Job drawing, mm, ordinate dimensions from the low corner. One solid piece. A direction names the side the tool comes from. Round coordinates to 2 decimals unless told otherwise and drop trailing zeros. Order: outer loops, then holes, each group sorted by start corner. A loop starts at its lowest first (then second) coordinate and runs counter-clockwise, first axis right, second up. Notation, with made-up numbers: (-1, 70.5) -> (42, 70.5) arc R22 cw to (42, 104.5) -> close; hole circle Ø3 at (1.5, -36). An arc over 180 degrees is marked (long way). Use CSV: the item, a comma, the result in double quotes.
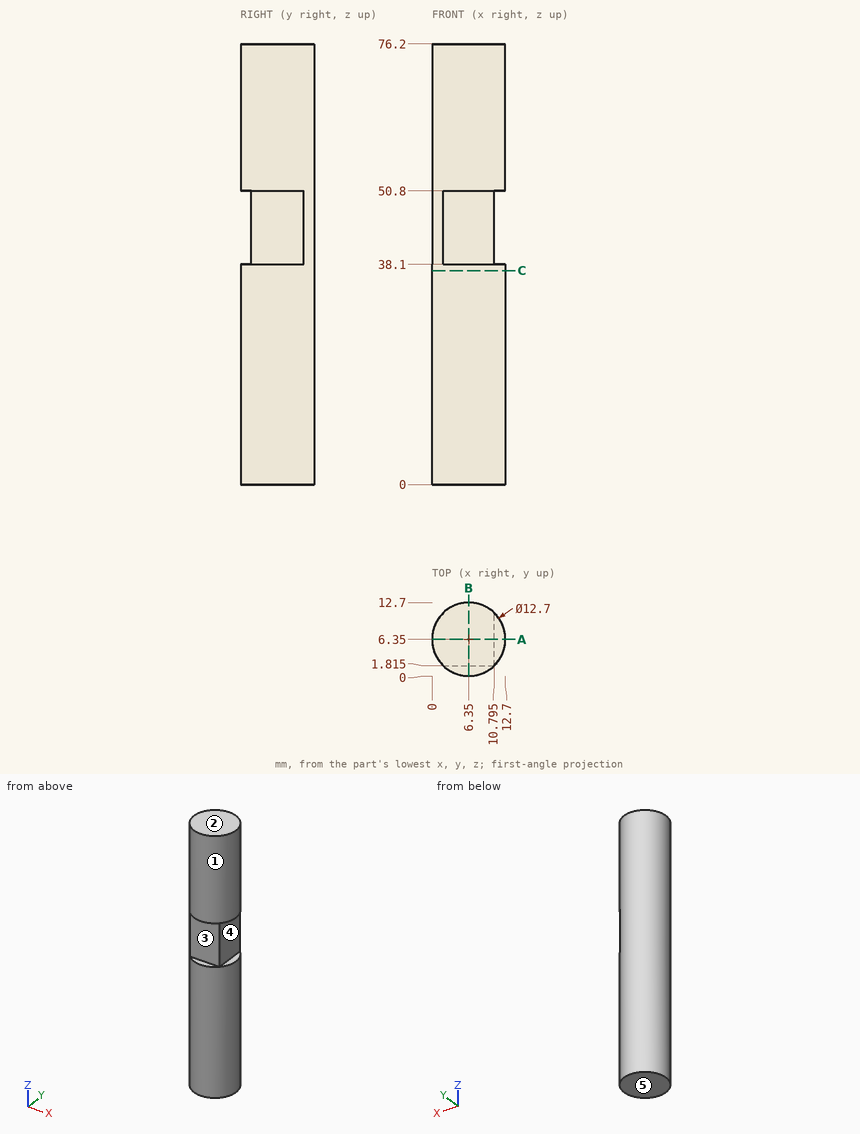
(1) Pull direction Z, two halves, no side cores. Call the marked faces 1, 2 and 3: released by +Z, released by -Z, zero draft, split by the parting line, or undercut.
Reply:
face 1,"zero draft"
face 2,"released by +Z"
face 3,"undercut"
(2) Cut at A-A, the plane y = 6.35. Give the cut face in (x, z) (3 decimals).
Reply:
outline,"(0, 0) -> (12.7, 0) -> (12.7, 38.1) -> (10.795, 38.1) -> (10.795, 50.8) -> (12.7, 50.8) -> (12.7, 76.2) -> (0, 76.2) -> close"
(3) Drop flat-ended pins along their axis: P1, Ø3, axis at y = 2.5, z = 30.5, coming from the -X side; P2, Ø4, axis at y = 3.5, z = 43.5, coming from the -X side; P3, Ø3, axis at y = 3, z = 13.5, coming from the +X side. Give the stop position or say it passes through.
Reply:
P1,"x = 0.45"
P2,"x = 0.06"
P3,"x = 12.42"
(4) Cut at C-C, the plane z = 37. Give the cut face in (x, y).
Reply:
outline,"circle Ø12.7 at (6.35, 6.35)"
(5) Cut at B-B, the plane x = 6.35. Give the cut face in (y, z) (1 decimal), then the cut area to 3 significant figures.
Reply:
outline,"(0, 0) -> (12.7, 0) -> (12.7, 76.2) -> (0, 76.2) -> (0, 50.8) -> (1.8, 50.8) -> (1.8, 38.1) -> (0, 38.1) -> close"
area,"945 mm2"
(6) Probe probe 1 along Z at (x, y) = (11.25, 3); probe 2 along Y at (x, z) = (6.75, 63); probe 3 along X at (y, z) = (6.25, 45.5) (1 decimal). List the from-to ranges inside material, lowest first. Write a range as [from, to].
Reply:
probe 1,"[0, 38.1], [50.8, 76.2]"
probe 2,"[0.01, 12.69]"
probe 3,"[0, 10.8]"
(7) Which spindle directions (+Z, -Z, +X, -X, +Y, -Y) get a long thin tool onto all of the face, cutting with end or side? Do the marked faces 4 and 5. Say none if no direction does.
Reply:
face 4,"+X, +Y, -Y"
face 5,"-Z, +X, -X, +Y, -Y"
